Autodesk Inventor part; units mm, degrees
ref_plane "Начальная плоскость" through (0, 0, 40) normal (0, 0, 1) x (1, 0, 0)
ref_plane "Конечная плоскость" through (0, 0, 200.17) normal (0, 0, 1) x (1, 0, 0)
ref_plane "РабПлоскость4" through (0, -158, 240.17) normal (0, 1, 0) x (1, 0, 0)
ref_plane "Начальная плоскость" through (0, 0, 40) normal (0, 0, 1) x (1, 0, 0)
ref_plane "Конечная плоскость" through (0, 0, 200.17) normal (0, 0, 1) x (1, 0, 0)
sketch "Эскиз" plane through (0, 0, 0) normal (0, 0, 1) x (1, 0, 0)
  line L0 (-1.43, 0) -> (-1.43, 40)
  line L1 (-1.43, 40) -> (43.57, 40)
  line L2 (43.57, 40) -> (43.57, 38.1774)
  line L3 (39.9881, 34.1993) -> (11.2338, 31.1771)
  line L4 (4.07, 23.221) -> (4.07, 0)
  line L5 (4.07, 0) -> (-1.43, 0) construction
  line L6 (23.82, 40) -> (23.82, 32.5) construction
  line L7 (43.57, 34.5758) -> (43.57, 32.5) construction
  line L8 (43.57, 32.5) -> (23.82, 32.5) construction
  line L9 (0, 15) -> (0, -27) construction
  line L10 (-5.539, 0) -> (16.0067, 0) construction
  line L11 (-1.43, 0) -> (-1.43, -40)
  line L12 (-1.43, -40) -> (43.57, -40)
  line L13 (43.57, -40) -> (43.57, -38.1774)
  line L14 (39.9881, -34.1993) -> (11.2338, -31.1771)
  line L15 (4.07, -23.221) -> (4.07, 0)
  arc A0 (11.2338, 31.1771) -> (4.07, 23.221) centre (12.07, 23.221) ccw
  arc A1 (4.07, -23.221) -> (11.2338, -31.1771) centre (12.07, -23.221) ccw
  arc A2 (39.9881, 34.1993) -> (43.57, 38.1774) centre (39.57, 38.1774) ccw
  arc A3 (43.57, -38.1774) -> (39.9881, -34.1993) centre (39.57, -38.1774) ccw
  line L16 (0, 56) -> (0, -56) construction
  line L17 (-15.5135, 0) -> (54.308, 0) construction
  point P0 (4.07, 30.4242)
  point P1 (43.57, -34.5758)
  point P2 (4.07, -30.4242)
  point P3 (23.82, -40)
  point P4 (23.82, -32.5)
  dimension "d0" = 5.5
  dimension "d1" = 40
  dimension "d2" = 45
  dimension "d3" = 7.5
  dimension "d4" = 19.75
  dimension "d5" = 2.0758
  dimension "d23" = 8
  dimension "d24" = 4
  dimension "d25" = 1.43
extrude "Тело" add sketch "Эскиз" along normal up to surface (160.17 mm away) from surface at 40
sketch "Sketch3" plane through (0, 0, 0) normal (0, 0, 1) x (1, 0, 0)
  line L0 (0, 0) -> (10, 0)
ref_plane "Work Plane3" through (0, 0, 0) normal (0, -1, 0) x (1, 0, 0)
sketch "Sketch4" plane through (0, 0, 0) normal (0, -1, 0) x (1, 0, 0)
  line L0 (-2, 40) -> (12, 40)
  line L1 (-2, 200.17) -> (12, 200.17)
  dimension "d29" = 160.17
ref_plane "РабПлоскость4" through (0, -158, 240.17) normal (0, 1, 0) x (1, 0, 0)
ref_plane "РабПлоскость5" through (0, 557.0652, 240.17) normal (0, 1, 0) x (1, 0, 0)
ref_plane "РабПлоскость6" through (0, 199.5326, 240.17) normal (0, 1, 0) x (1, 0, 0)
sketch "Эскиз5" plane through (0, 199.5326, 240.17) normal (0, 1, 0) x (1, 0, 0)
  line L0 (-1.43, 0) -> (-1.43, 40)
  line L1 (-1.43, 40) -> (43.57, 40)
  line L2 (43.57, 40) -> (43.57, 38.1774)
  arc A0 (39.9881, 34.1993) -> (43.57, 38.1774) centre (39.57, 38.1774) ccw
  line L3 (39.9881, 34.1993) -> (11.2338, 31.1771)
  arc A1 (11.2338, 31.1771) -> (4.07, 23.221) centre (12.07, 23.221) ccw
  line L4 (4.07, 23.221) -> (4.07, 0)
  line L5 (4.07, -23.221) -> (4.07, 0)
  arc A2 (4.07, -23.221) -> (11.2338, -31.1771) centre (12.07, -23.221) ccw
  line L6 (39.9881, -34.1993) -> (11.2338, -31.1771)
  arc A3 (43.57, -38.1774) -> (39.9881, -34.1993) centre (39.57, -38.1774) ccw
  line L7 (43.57, -40) -> (43.57, -38.1774)
  line L8 (-1.43, -40) -> (43.57, -40)
  line L9 (-1.43, 0) -> (-1.43, -40)
extrude "Выдавливание2" add sketch "Эскиз5" along normal up to surface (715.0652 mm away) from surface at -357.5326 separate body
feature "Комбинировать1" [suppressed]
ref_plane "РабПлоскость7" through (0, 562.5, 0) normal (0, -1, 0) x (1, 0, 0)
ref_plane "РабПлоскость8" through (0, -158, 0) normal (0, -1, 0) x (1, 0, 0)
ref_plane "РабПлоскость9" through (0, 202.25, 0) normal (0, -1, 0) x (1, 0, 0)
sketch "Эскиз6" plane through (0, 202.25, 0) normal (0, -1, 0) x (1, 0, 0)
  line L0 (-1.43, 0) -> (-1.43, 40)
  line L1 (-1.43, 40) -> (43.57, 40)
  line L2 (43.57, 40) -> (43.57, 38.1774)
  arc A0 (39.9881, 34.1993) -> (43.57, 38.1774) centre (39.57, 38.1774) ccw
  line L3 (39.9881, 34.1993) -> (11.2338, 31.1771)
  arc A1 (11.2338, 31.1771) -> (4.07, 23.221) centre (12.07, 23.221) ccw
  line L4 (4.07, 23.221) -> (4.07, 0)
  line L5 (4.07, -23.221) -> (4.07, 0)
  arc A2 (4.07, -23.221) -> (11.2338, -31.1771) centre (12.07, -23.221) ccw
  line L6 (39.9881, -34.1993) -> (11.2338, -31.1771)
  arc A3 (43.57, -38.1774) -> (39.9881, -34.1993) centre (39.57, -38.1774) ccw
  line L7 (43.57, -40) -> (43.57, -38.1774)
  line L8 (-1.43, -40) -> (43.57, -40)
  line L9 (-1.43, 0) -> (-1.43, -40)
extrude "Выдавливание3" add sketch "Эскиз6" along normal up to surface (720.5 mm away) from surface at -360.25 separate body
feature "Комбинировать2" [suppressed]
ref_plane "РабПлоскость10" through (-1.43, -158, 200.17) normal (0, 0, 1) x (1, 0, 0)
split "Разделение1" plane through (-1.43, -158, 200.17) removes the side toward (0, 0, 1)
ref_plane "РабПлоскость11" through (-1.43, 562.5, 40) normal (0, 0, -1) x (-1, 0, 0)
split "Разделение2" plane through (-1.43, 562.5, 40) removes the side toward (0, 0, -1)
equation "\"d0\" = G_T"
equation "\"d1\" = 0.5 * G_H"
equation "\"d2\" = G_W"
equation "\"d3\" = G_T1"
equation "\"d4\" = G_C"
equation "\"d23\" = G_IR"
equation "\"d24\" = G_ER"
equation "\"d25\" = ex"
equation "\"d6\" = G_L"
equation "\"G_W\" = 45"
equation "\"G_T\" = 5.5"
equation "\"G_T1\" = 7.5"
equation "\"G_NG\" = 0.105104"
equation "\"G_ER\" = 4"
equation "\"G_IR\" = 8"
equation "\"G_C\" = 19.75"
equation "\"G_L\" = d29"
equation "\"ex\" = 1.43"
equation "\"d27\" = G_OFFSET_END + B_L"
equation "\"B_L\" = 240.17"
properties part number "ISO 657/11 - CH 80 x 8 - 160,17" material "Сталь, мягкая"
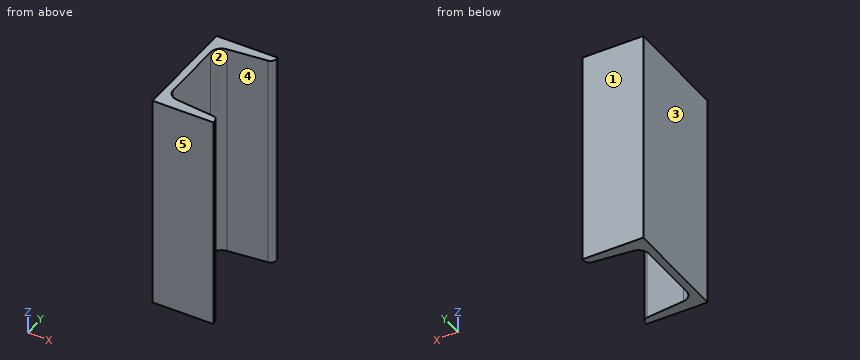
The listing builds one solid part. Answer for the finished solid, in the listing's coordinates (mm). Face numbers are marked on the shaded views. A direction names the side the tool comes from. Give positions to 0.01 mm unless a question says otherwise; leave off trailing zeros. Order: outer loops, then holes, each group sorted by start corner. A loop starts at its lowest first (then second) coordinate and runs counter-clockwise, first axis right, second up. Notation, with made-up numbers: (-19.5, 28) - (-12.5, 28) arc R16 cw to (-12.5, 55) - close; hole circle Ø2 at (0, -0.75). An arc over 180 degrees is marked (long way). Answer in a Markdown table with one row per item. Add a question column.
Q1. For a pull along Y with two mould halves and no side action, classify the marked faces 3, 4 and 5 as released by +Y, released by -Y, zero draft, split by the parting line, or undercut.
Q2. Given P1, Ø8, axis at y = -9.5, z = 83.5, coming from the +X side, flat-ended and moving along its own axis, determine where the tip first touches the part or whether it passes through.
Q3. The part is cut by section A-A (z = 138). Determine the outline of the cut face in (x, y).
Q4. The part is cut by section D-D (x = 22.5). Determine the outline of the cut face in (y, z), then the cut area to 3 significant figures.
Q5. The part is cut by section B-B (x = 8). Determine the outline of the cut face in (y, z).
Q6. Find the intervals of material crossed by line 1 along X through (y, z) = (-18, 94); line 2 along Y through (x, z) = (41, 97.5); line 3 along Y through (x, z) = (15, 75.5), in increasing order. Write a range as [from, to].
Q7. The part is cut by section C-C (y = -11.5). Determine the outline of the cut face in (x, z), then the cut area to 3 significant figures.
Q8. Which of the six approach directions +Z, -Z, +X, -X, +Y, -Y give full straight-line access (tool end or side, diameter ignored) to the marked faces 1 and 2?
Determined:
| question | item | result |
|---|---|---|
| 1 | face 3 | zero draft |
| 1 | face 4 | undercut |
| 1 | face 5 | released by -Y |
| 2 | P1 | stops at x = 4.07 |
| 3 | outline | (-1.43, -40) - (43.57, -40) - (43.57, -38.18) arc R4 ccw to (39.99, -34.2) - (11.23, -31.18) arc R8 cw to (4.07, -23.22) - (4.07, 23.22) arc R8 cw to (11.23, 31.18) - (39.99, 34.2) arc R4 ccw to (43.57, 38.18) - (43.57, 40) - (-1.43, 40) - close |
| 4 | outline | (-40, 40) - (-32.36, 40) - (-32.36, 200.17) - (-40, 200.17) - close; (32.36, 40) - (40, 40) - (40, 200.17) - (32.36, 200.17) - close |
| 4 | area | 2,450 mm² |
| 5 | outline | (-40, 40) - (-30.11, 40) - (-30.11, 200.17) - (-40, 200.17) - close; (30.11, 40) - (40, 40) - (40, 200.17) - (30.11, 200.17) - close |
| 6 | line 1 | x = [-1.43, 4.07] |
| 6 | line 2 | y = [-40, -34.44], [34.44, 40] |
| 6 | line 3 | y = [-40, -31.57], [31.57, 40] |
| 7 | outline | (-1.43, 40) - (4.07, 40) - (4.07, 200.17) - (-1.43, 200.17) - close |
| 7 | area | 881 mm² |
| 8 | face 1 | +Z, -Z, +X, -X, +Y |
| 8 | face 2 | +Z, -Z, +X |
